from build123d import *

# Parameters (mm, degrees)
F1_DEPTH = 19.05
F2_W     = 44.45
F2_H     = 19.05
F3_DEPTH = 63.5
F5_DEPTH = 19.05


with BuildPart() as f1:
    # F0 (on Right) → F1 (new body)
    with BuildSketch(Plane.YZ):
        Polygon((0.958807, 20.364464), (-43.491193, -11.385536), (-43.491193, -24.085536), (20.008807, -24.085536), (20.008807, 20.364464), align=None)
    extrude(amount=F1_DEPTH)

    # F2 (on face) → F3 (join)
    with BuildSketch(Plane(origin=(0, 0, 0), x_dir=(0, -1, 0), z_dir=(-1, 0, 0))):
        with Locations((2.216193, -14.560536)):
            Rectangle(F2_W, F2_H)
    extrude(amount=F3_DEPTH)

    # F4 (on face) → F5 (join)
    with BuildSketch(Plane(origin=(-63.5, 0, 0), x_dir=(0, -1, 0), z_dir=(-1, 0, 0))):
        Polygon((24.441193, -5.035536), (24.441193, -24.085536), (43.491193, -24.085536), (43.491193, -11.385536), (0, 20.364464), (-19.05, 20.364464), (-19.59789, -5.035536), align=None)
        Polygon((-19.59789, -5.035536), (-20.008807, -24.085536), (24.441193, -24.085536), (24.441193, -5.035536), align=None)
    extrude(amount=F5_DEPTH)


solid = f1.part
Source: CAD feature listing. Evaluate the final solid. Frame: model axes, mm. A direction names the side the tool comes from. Round coordinates to 2 decimals unless told otherwise and drop trailing zeros. Write each loop counter-clockwise with the first axis right and the second up, starting at its lowest first coordinate (ties: lowest second). Pieces come first, ordered by that corner, then holes. Notation, with made-up numbers: M 4,46 L 27,46 A17 cw 27,79 Z; hole C 44.25,85 d3. An arc over 180 degrees is marked long. One line per item, written item: value. Start each with the question number.
Item 1: Ray query, L1, parallel to X at y = 6, z = 16.5; L2, parallel to Z at x = -19, y = -5; L3, parallel to Y at x = -19, z = -21. Return the intervals inside material, ascending. Write a range as from..to.
Item 2: Section query D-D (y = -29). Return the cut outline in (x, z).
Item 3: Section query B-B (z = 17.5). Return the cut outline in (x, y), plus the area to 3 significant figures.
Item 4: Section query C-C (x = 7). Return the cut outline in (y, z), plus the area to 3 significant figures.
Item 5: Section query A-A (y = 5). Return the cut outline in (x, z), plus the area to 3 significant figures.
Item 6: Mould query, pull axis X, two halves, no side actions, for faces 4 (the flat face through (-82.55, -4, -6)), 5 (the flat face through (-31, -24.441, -15)), 6 (the flat face through (19.05, -5, -6)), 7 (the flat face through (9, -43.491, -18)). Classes: pulls with the +X half, pulls with the -X half, needs draft (parallel to the pull), parting line crosses it, or undercut.
Item 7: Pin query (flat end, axial travel): pin 1 (15 mm diameter, centred on x = -41, z = -12, fed in from -Y); pin 2 (5 mm diameter, centred on x = -49.5, z = -2.5, fed in from -Y); pin 3 (3 mm diameter, centred on x = -46.5, y = 11, fed in from +Z). Return the tip coordinate at first contact, or that it passes through.
Item 8: Set-up query: faces 1 (the flat face through (9.39, -20.96, 4.71)), 2 (the flat face through (-63.5, -12, -2)), 3 (the flat face through (-31, -2, -5.036)). Return all of +Z, -Z, +X, -X, +Y, -Y with unobstructed straight access to the full face (end or side cutting, diameter ignored); none if empty.
Result set:
1. L1: x = -82.55..-63.5, 0..19.05
1. L2: z = -24.09..-5.04
1. L3: y = -24.44..20.01
2. outline: M -82.55,-24.09 L -63.5,-24.09 L -63.5,-0.81 L -82.55,-0.81 Z; M 0,-24.09 L 19.05,-24.09 L 19.05,-1.03 L 0,-1.03 Z
3. outline: M -82.55,-3.92 L -63.5,-3.92 L -63.5,19.11 L -82.55,19.11 Z; M 0,-3.05 L 19.05,-3.05 L 19.05,20.01 L 0,20.01 Z
3. area: 878 mm²
4. outline: M -43.49,-24.09 L 20.01,-24.09 L 20.01,20.36 L 0.96,20.36 L -43.49,-11.39 Z
4. area: 2,120 mm²
5. outline: M -82.55,-24.09 L 19.05,-24.09 L 19.05,20.36 L 0,20.36 L 0,-5.04 L -63.5,-5.04 L -63.5,20.36 L -82.55,20.36 Z
5. area: 2,900 mm²
6. face 4: pulls with the -X half
6. face 5: undercut
6. face 6: pulls with the +X half
6. face 7: needs draft
7. pin 1: stops at y = -24.44
7. pin 2: passes through
7. pin 3: stops at z = -5.04
8. face 1: +Z, +X, -Y
8. face 2: +Z, -Y
8. face 3: +Z, +Y, -Y
